```python
from build123d import *

# Parameters (mm, degrees)
F1_DEPTH = 6.35
F2_W     = 91.44
F2_H     = 100.33
F3_DEPTH = 1.524
F5_DEPTH = 5.334
F6_DEPTH = 6.35


with BuildPart() as f1:
    # F0 (on Front) → F1 (new body)
    with BuildSketch(Plane.XZ):
        Polygon((12.5022814354, 76.191857674), (-45.9177185646, 76.191857674), (-56.0777185646, 66.031857674), (-56.0777185646, -13.978142326), (-45.9177185646, -24.138142326), (12.5022814354, -24.138142326), (22.6622814354, -13.978142326), (22.6622814354, 66.031857674), align=None)
        Polygon((-54.5537185646, 65.4005962049), (-45.2864570956, 74.667857674), (11.8710199663, 74.667857674), (21.1382814354, 65.4005962049), (21.1382814354, -13.346880857), (11.8710199663, -22.614142326), (-45.2864570956, -22.614142326), (-54.5537185646, -13.346880857), align=None, mode=Mode.SUBTRACT)
    extrude(amount=F1_DEPTH)

    # F2 (on face) → F3 (join)
    with BuildSketch(Plane(origin=(0, 0, 0), x_dir=(-1, 0, 0), z_dir=(0, 1, 0))):
        with Locations((16.7077185646, 26.026857674)):
            Rectangle(F2_W, F2_H)
    extrude(amount=F3_DEPTH)

    # F4 (on face) → F5 (cut, symmetric)
    with BuildSketch(Plane.XZ):
        Polygon((11.8710199663, 74.667857674), (-45.2864570956, 74.667857674), (-54.5537185646, 65.4005962049), (-54.5537185646, -13.346880857), (-45.2864570956, -22.614142326), (11.8710199663, -22.614142326), (21.1382814354, -13.346880857), (21.1382814354, 65.4005962049), align=None)
    extrude(amount=F5_DEPTH, both=True, mode=Mode.SUBTRACT)

    # F0 (on Front) → F6 (join)
    with BuildSketch(Plane.XZ):
        Polygon((12.5022814354, 76.191857674), (-45.9177185646, 76.191857674), (-56.0777185646, 66.031857674), (-56.0777185646, -13.978142326), (-45.9177185646, -24.138142326), (12.5022814354, -24.138142326), (22.6622814354, -13.978142326), (22.6622814354, 66.031857674), align=None)
        Polygon((-54.5537185646, 65.4005962049), (-45.2864570956, 74.667857674), (11.8710199663, 74.667857674), (21.1382814354, 65.4005962049), (21.1382814354, -13.346880857), (11.8710199663, -22.614142326), (-45.2864570956, -22.614142326), (-54.5537185646, -13.346880857), align=None, mode=Mode.SUBTRACT)
    extrude(amount=F6_DEPTH)


solid = f1.part
```
Geometry check sheet. Reference: the model listing, model coordinates, mm. A direction names the side the tool comes from. Coordinates: 2 decimals unless noted, no trailing zeros. Order: outer loops, then holes, each group sorted by start corner. A loop starts at its lowest first (then second) coordinate and runs counter-clockwise, first axis right, second up. Notation, with made-up numbers: (-21, 20.25) - (-13, 20.25) arc R30 ccw to (-13, 56.25) - close; hole circle Ø10 at (56, 39.5). An arc over 180 degrees is marked (long way). Answer in a Markdown table with one row per item. Add a question column.
1. Gauge pin test, flat ends, axial feed: pin 1 Ø4 at (y, z) = (-3.5, 20.5) entering from +X; pin 2 Ø1.9 at (y, z) = (-3, 30) entering from -X. Record the tip position at first contact, or that the pin passes through.
2. Section check B-B (z = 28). Enter the section's corners in (x, y).
3. Section check A-A (y = -3.5). Enter the section's corners in (x, z), plus the area to 3 significant figures.
4. Draft check along X on faces 1 (the face through (24, 1.524, 23)), 2 (the face through (-16, -2, 74.668)), 3 (the face through (22.662, -3, 25)). Enter one of: +X half, -X half, draft (parallel to the pull), parting line (faces both ways), or undercut.
5. Material ranges on L1, parallel to X at y = -2.5, z = 42; L2, parallel to X at y = 0.25, z = 11.5; L3, parallel to Z at x = 11, y = 1.25, recorded low to high. Write a range as [from, to].
6. Section check C-C (x = -44). Enter the section's corners in (y, z).
7. Access from +Z, -Z, +X, -X, +Y, -Y to the whole of each face (thin tool, end or side, straight path). Record for faces 4 (the face through (-17, -2, -22.614)), 5 (the face through (17.653, -3.131, 71.041)), 6 (the face through (17.51, -3.13, -19.13)), 7 (the face through (-51.069, -3.131, -18.987)).
Data:
| question | item | result |
|---|---|---|
| 1 | pin 1 | stops at x = 22.66 |
| 1 | pin 2 | stops at x = -56.08 |
| 2 | outline | (-62.43, 0) - (-56.08, 0) - (-56.08, -6.35) - (-54.55, -6.35) - (-54.55, 1.52) - (-62.43, 1.52) - close; (21.14, -6.35) - (22.66, -6.35) - (22.66, 0) - (29.01, 0) - (29.01, 1.52) - (21.14, 1.52) - close |
| 3 | outline | (-56.08, -13.98) - (-45.92, -24.14) - (12.5, -24.14) - (22.66, -13.98) - (22.66, 66.03) - (12.5, 76.19) - (-45.92, 76.19) - (-56.08, 66.03) - close; hole (-54.55, -13.35) - (-45.29, -22.61) - (11.87, -22.61) - (21.14, -13.35) - (21.14, 65.4) - (11.87, 74.67) - (-45.29, 74.67) - (-54.55, 65.4) - close |
| 3 | area | 502 mm² |
| 4 | face 1 | draft |
| 4 | face 2 | undercut |
| 4 | face 3 | +X half |
| 5 | L1 | x = [-56.08, -54.55], [21.14, 22.66] |
| 5 | L2 | x = [-62.43, -54.55], [21.14, 29.01] |
| 5 | L3 | z = [-24.14, -22.61], [74.67, 76.19] |
| 6 | outline | (-6.35, -24.14) - (1.52, -24.14) - (1.52, -22.61) - (-6.35, -22.61) - close; (-6.35, 74.67) - (1.52, 74.67) - (1.52, 76.19) - (-6.35, 76.19) - close |
| 7 | face 4 | +Y, -Y |
| 7 | face 5 | +Z, +X, -Y |
| 7 | face 6 | -Z, +X, -Y |
| 7 | face 7 | -Z, -X, -Y |
